from build123d import *

# Parameters (mm, degrees)
F0_W     = 1219.2
F0_H     = 609.6
F1_DEPTH = 457.2
F2_T     = -12.7
F4_DEPTH = 444.5


with BuildPart() as f1:
    # F0 (on Top) → F1 (new body)
    with BuildSketch(Plane.XY):
        with Locations((4.2110532522, -30.9912272245)):
            Rectangle(F0_W, F0_H)
    extrude(amount=F1_DEPTH)

    # F2
    f2_openings = [f1.faces().sort_by_distance(p)[0] for p in [
        (4.211053, -30.991227, 457.2),
    ]]
    offset(amount=F2_T, openings=f2_openings)

    # F3 (on face) → F4 (join, through all)
    with BuildSketch(Plane.XY.offset(12.7)):
        Polygon((-465.6889467478, 210.3087727755), (-592.6889467478, 210.3087727755), (-592.6889467478, 197.6087727755), (601.1110532522, 197.6087727755), (601.1110532522, 210.3087727755), (474.1110532522, 210.3087727755), (474.1110532522, 261.1087727755), (461.4110532522, 261.1087727755), (461.4110532522, 210.3087727755), (-452.9889467478, 210.3087727755), (-452.9889467478, 261.1087727755), (-465.6889467478, 261.1087727755), align=None)
    extrude(amount=F4_DEPTH)


solid = f1.part
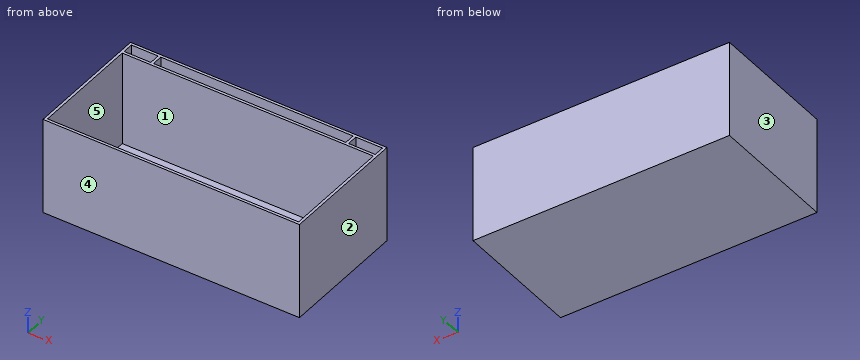
The listing builds one solid part. Answer for the finished solid, in the listing's coordinates (mm). Face numbers are marked on the shaded views. A direction names the side the tool comes from. Coordinates: 2 decimals unless noted, no trailing zeros. Order: outer loops, then holes, each group sorted by start corner. A loop starts at its lowest first (then second) coordinate and runs counter-clockwise, first axis right, second up. Notation, with made-up numbers: (-8.75, 56) -> (47.25, 56) arc R24 cw to (47.25, 93) -> close; hole circle Ø3 at (-1.75, 8). An arc over 180 degrees is marked (long way). Answer in a Markdown table with one row per item. Add a question column.
Item 1: Find the intervals of material crossed by L1, parallel to X at y = 225, z = 269; L2, parallel to Y at x = 229, z = 208; L3, parallel to Y at x = -456, z = 265.5, in increasing order. Write a range as from..to.
Item 2: Find section C-C (y = 97). Write down the section's boundary in (x, z), then the cut area to 3 significant figures.
Item 3: This flat-tipped pin is pushed along its axis until it touches: P1, Ø8, axis at x = -350, y = -108, coming from the +Z side. Where does it stop, or does it pass through?
Item 4: Determine the mould class of the marked faces 3, 4 and 5 for opening direction Y: +Y half, -Y half, draft (parallel to the pull), parting line (faces both ways), or undercut.
Item 5: Find section B-B (x = -67). Write down the section's boundary in (y, z).
Item 6: Find section A-A (z = 412.5). Write down the section's boundary in (x, y).
Item 7: Which of the six approach directions +Z, -Z, +X, -X, +Y, -Y give full straight-line access (tool end or side, diameter ignored) to the marked faces 1 and 2?
Result set:
| question | item | result |
|---|---|---|
| 1 | L1 | x = -605.39..-592.69, -465.69..-452.99, 461.41..474.11, 601.11..613.81 |
| 1 | L2 | y = -335.79..-323.09, 197.61..210.31, 261.11..273.81 |
| 1 | L3 | y = -335.79..-323.09, 197.61..273.81 |
| 2 | outline | (-605.39, 0) -> (613.81, 0) -> (613.81, 457.2) -> (601.11, 457.2) -> (601.11, 12.7) -> (-592.69, 12.7) -> (-592.69, 457.2) -> (-605.39, 457.2) -> close |
| 2 | area | 26,800 mm² |
| 3 | P1 | stops at z = 12.7 |
| 4 | face 3 | draft |
| 4 | face 4 | -Y half |
| 4 | face 5 | undercut |
| 5 | outline | (-335.79, 0) -> (273.81, 0) -> (273.81, 457.2) -> (261.11, 457.2) -> (261.11, 12.7) -> (210.31, 12.7) -> (210.31, 457.2) -> (197.61, 457.2) -> (197.61, 12.7) -> (-323.09, 12.7) -> (-323.09, 457.2) -> (-335.79, 457.2) -> close |
| 6 | outline | (-605.39, -335.79) -> (613.81, -335.79) -> (613.81, 273.81) -> (-605.39, 273.81) -> close; hole (-592.69, -323.09) -> (601.11, -323.09) -> (601.11, 197.61) -> (-592.69, 197.61) -> close; hole (-592.69, 210.31) -> (-465.69, 210.31) -> (-465.69, 261.11) -> (-592.69, 261.11) -> close; hole (-452.99, 210.31) -> (461.41, 210.31) -> (461.41, 261.11) -> (-452.99, 261.11) -> close; hole (474.11, 210.31) -> (601.11, 210.31) -> (601.11, 261.11) -> (474.11, 261.11) -> close |
| 7 | face 1 | +Z |
| 7 | face 2 | +Z, -Z, +X, +Y, -Y |
